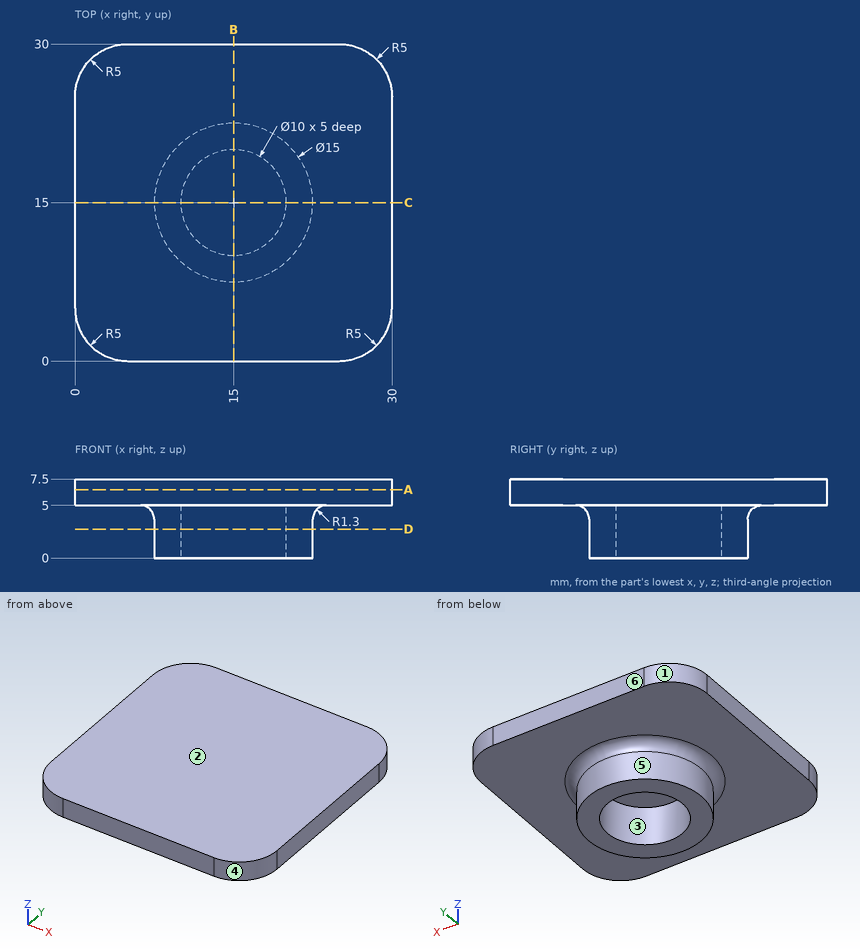
Could you check a few things on this drawing? It's one solid part, dimensions in mm from its lowest x, y, z. A direction names the side the tool comes from. Coordinates: 2 decimals unless noted, no trailing zeros. Write each loop counter-clockwise with the first axis right and the second up, starting at its lowest first coordinate (ties: lowest second). Pieces come first, ordered by that corner, then holes.
Q1. Imagine slicing it at A-A, the plane z = 6.5. List the corners of the cut face in (x, y) for me.
Results found:
outline: (0, 5) arc R5 ccw to (5, 0) - (25, 0) arc R5 ccw to (30, 5) - (30, 25) arc R5 ccw to (25, 30) - (5, 30) arc R5 ccw to (0, 25) - close
Q2. Imagine slicing it at B-B, the plane x = 15. List the corners of the cut face in (y, z) for me, plus the area to 3 significant figures.
Results found:
outline: (0, 5) - (6.2, 5) arc R1.3 cw to (7.5, 3.7) - (7.5, 0) - (10, 0) - (10, 5) - (20, 5) - (20, 0) - (22.5, 0) - (22.5, 3.7) arc R1.3 cw to (23.8, 5) - (30, 5) - (30, 7.5) - (0, 7.5) - close
area: 101 mm2
Q3. If we mould it in two halves opening along X, with no side actions, what happens to the marked faces 1, 2, 3 and 4? For each: +X half, -X half, draft (parallel to the pull), parting line (faces both ways), or undercut.
Results found:
face 1: -X half
face 2: draft
face 3: undercut
face 4: +X half
Q4. Imagine slicing it at D-D, the plane z = 2.75. List the corners of the cut face in (x, y) for me.
Results found:
outline: circle Ø15 at (15, 15); hole circle Ø10 at (15, 15)
Q5. For P1, Ø2, axis at y = 27, z = 3.5, coming from the -X side; P2, Ø5, axis at x = 13, y = 16, coming from the -Z side; P3, Ø2, axis at y = 22, z = 1.5, coming from the -X side; P4, Ø1.5, axis at y = 22, z = 1, coming from the -X side, each with a flat end and sliding along its axis, tell me the tip position at first contact or that it passes through.
Results found:
P1: passes through
P2: stops at z = 5
P3: stops at x = 10.5
P4: stops at x = 10.85
Q6. Which directions (+Z, -Z, +X, -X, +Y, -Y) give clear straight access to the entire face, cutting with the end or side of a thin tool? Please do the marked faces 5 and 6.
Results found:
face 5: -Z
face 6: +Z, -Z, +X, -X, +Y
Q7. Please list where these lines run through material, in increasing order: L1, parallel to Y at x = 15, z = 3.2; L2, parallel to Z at x = 23.5, y = 21.5; L3, parallel to X at y = 13, z = 1.75.
Results found:
L1: y = 7.5 to 10, 20 to 22.5
L2: z = 5 to 7.5
L3: x = 7.77 to 10.42, 19.58 to 22.23
